from build123d import *

# Parameters (mm, degrees)
RESSALTO_EXTRUS_O1_DEPTH = 5


with BuildPart() as part:
    # Esboço1 → Ressalto-extrusão1 (new body)
    with BuildSketch(Plane.XY):
        with BuildLine():
            Line((0, -6.5), (19.621320344, -6.5))
            ThreePointArc((19.621320344, -6.5), (20.545199876, -5.882683432), (20.328427125, -4.792893219))
            Line((20.328427125, -4.792893219), (13.767766953, 1.767766953))
            Line((13.767766953, 1.767766953), (12, 0))
            Line((12, 0), (14.292893219, -2.292893219))
            ThreePointArc((14.292893219, -2.292893219), (14.50966597, -3.382683432), (13.585786438, -4))
            Line((13.585786438, -4), (0, -4))
            ThreePointArc((0, -4), (-3.731407445, 1.441040764), (2.688555117, 2.961700759))
            Line((2.688555117, 2.961700759), (4.457591724, 4.730737366))
            ThreePointArc((4.457591724, 4.730737366), (-6.041514416, 2.397937356), (0, -6.5))
        make_face()
    extrude(amount=RESSALTO_EXTRUS_O1_DEPTH)


solid = part.part
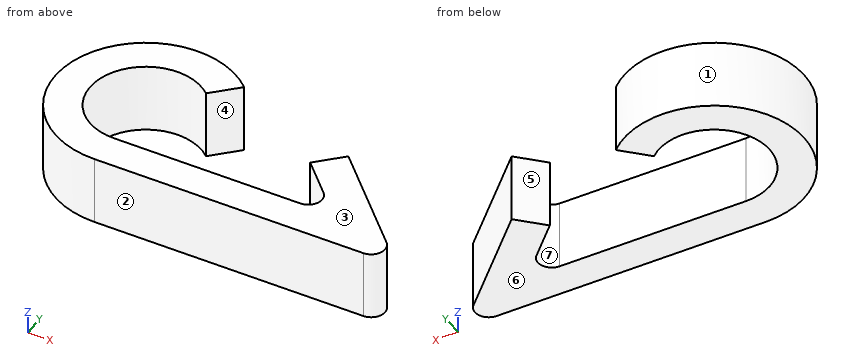
Geometry check sheet. Reference: the model listing, model coordinates, mm. Face numbers are marked on the shaded views. A direction names the side the tool comes from. Round coordinates to 2 decimals unless told otherwise and drop trailing zeros. Loops run counter-clockwise (first coordinate to the right, second up) from the corner with the lowest first, then second, coordinate; pieces in that order, holes last. Notation, with made-up numbers: (7, 38) - (13, 38) arc R28 cw to (13, 75) - close; hole circle Ø6 at (50.25, 44). An arc over 180 degrees is marked (long way). One line per question, with ' | ' between items. Start each with the question number.
1. Cross-section at A-A on x = -0.25. Record the cut outline in (y, z).
2. Cross-section at B-B on z = 1.7. Record the cut outline in (x, y), then the cut area to 3 significant figures.
3. Scan lines: line 1 (Y direction, x = 0, z = 1.45); line 2 (X direction, y = 0.75, z = 3.55); line 3 (X direction, y = -0.25, z = 2.85). Record each from-to range of solid material in increasing order. Write a range as [from, to].
4. Cross-section at C-C on y = -1. Record the cut outline in (x, z).
5. Tool access check on the marked faces 5, 6 and 7. Record the directions out of +Z, -Z, +X, -X, +Y, -Y that give a thin tool (end or side, any length) a straight path to the whole face; none if there is none.
6. Depth check by flat-ended pin: pin 1 (1.5 mm diameter, centred on y = -4, z = 2, fed in from -X). Enter the tip coordinate at first touch or a pass-through.
7. Draft check along Y on the marked faces 1, 2, 3 and 4. Enter one of: released by +Y, released by -Y, zero draft, split by the parting line, or undercut.
8. Cross-section at D-D on x = 5. Record the cut outline in (y, z), then the cut area to 3 significant figures.
Taken from the geometry:
1) outline: (-6.5, 0) - (-3.99, 0) - (-3.99, 5) - (-6.5, 5) - close; (3.99, 0) - (6.5, 0) - (6.5, 5) - (3.99, 5) - close
2) outline: (0, -6.5) - (19.62, -6.5) arc R1 ccw to (20.33, -4.79) - (13.77, 1.77) - (12, 0) - (14.29, -2.29) arc R1 cw to (13.59, -4) - (0, -4) arc R4 cw (long way) to (2.69, 2.96) - (4.46, 4.73) arc R6.5 ccw (long way) to start | area: 120 mm²
3) line 1: [-6.5, -4], [4, 6.5] | line 2: [-6.46, -3.93], [12.75, 14.79] | line 3: [-6.5, -3.99], [12.25, 15.79]
4) outline: (-6.42, 0) - (-3.87, 0) - (-3.87, 5) - (-6.42, 5) - close; (13, 0) - (16.54, 0) - (16.54, 5) - (13, 5) - close
5) face 5: +Z, -Z, +Y | face 6: -Z, +X, -X, +Y, -Y | face 7: +Z, -Z
6) pin 1: x = -5.63
7) face 1: split by the parting line | face 2: released by -Y | face 3: zero draft | face 4: undercut
8) outline: (-6.5, 0) - (-4, 0) - (-4, 5) - (-6.5, 5) - close | area: 12.5 mm²
